For this review, use the dimensioned drawing (mm, ordinates from the lowest corner) and the shaded views. Round coordinates to 2 decimals unless told otherwise and drop trailing zeros. Write each loop counter-clockwise with the first axis right and the second up, starting at its lowest first coordinate (ties: lowest second). Pieces come first, ordered by that corner, then holes.
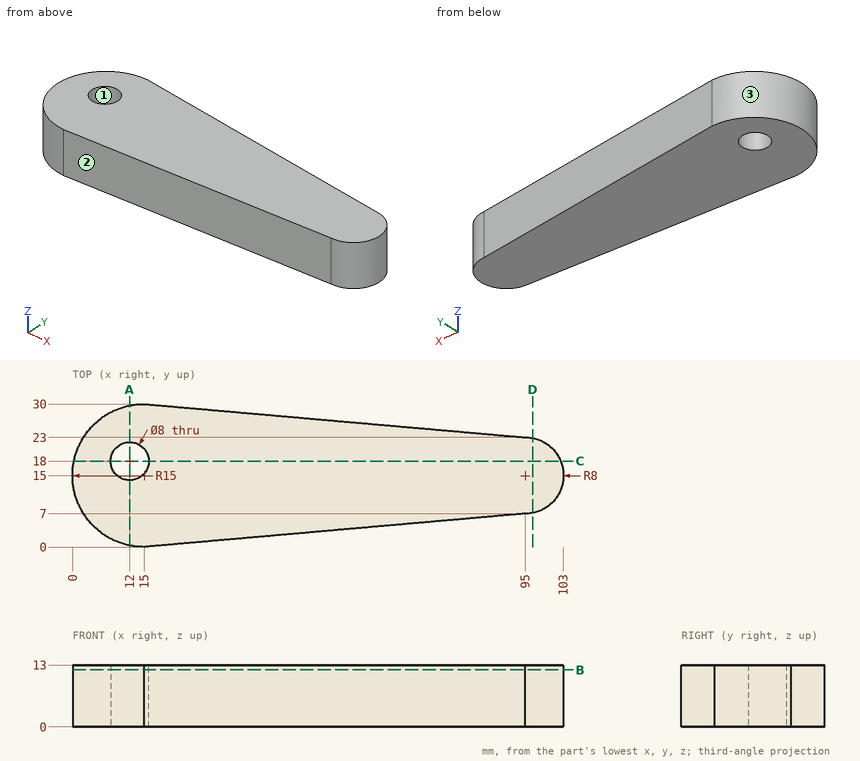
1) Add section C-C on y = 18. State the section outline as (x, z) points, and give its area (3 significant figures).
2) Add section A-A on x = 12. State the section outline as (y, z) points.
3) For line 1 along Y through (x, z) = (12, 7.25); line 2 along X through (y, z) = (18, 9.5); line 3 along X through (y, z) = (16.75, 4.75), list the stretches that pass through material, from the lowest coordinate up.
4) For P1, Ø2, axis at y = 20.5, z = 2.5, coming from the +X side; P2, Ø1, axis at y = 20, z = 6.5, coming from the -X side, all flat-tipped, find the tip position at first contact; note any pin that passes through.
5) Add section B-B on z = 12. State the section outline as (x, y) points, and give its area (3 significant figures).
6) The part is to be moulded in two halves that separate along X. For the marked faces 1, 2 and 3, say which applies: pulls with the +X half, pulls with the -X half, needs draft (parallel to the pull), parting line crosses it, or undercut.
7) Add section D-D on x = 96.5. State the section outline as (y, z) points, and give its area (3 significant figures).
Computed:
1. outline: (0.3, 0) - (8, 0) - (8, 13) - (0.3, 13) - close; (16, 0) - (102.42, 0) - (102.42, 13) - (16, 13) - close
1. area: 1,220 mm2
2. outline: (0.3, 0) - (14, 0) - (14, 13) - (0.3, 13) - close; (22, 0) - (29.7, 0) - (29.7, 13) - (22, 13) - close
3. line 1: y = 0.3 to 14, 22 to 29.7
3. line 2: x = 0.3 to 8, 16 to 102.42
3. line 3: x = 0.1 to 8.2, 15.8 to 102.81
4. P1: stops at x = 101.61
4. P2: stops at x = 0.69
5. outline: (15, 0) - (95, 7) arc R8 ccw to (95, 23) - (15, 30) arc R15 ccw to start; hole circle Ø8 at (12, 18)
5. area: 2,240 mm2
6. face 1: undercut
6. face 2: pulls with the +X half
6. face 3: pulls with the -X half
7. outline: (7.14, 0) - (22.86, 0) - (22.86, 13) - (7.14, 13) - close
7. area: 204 mm2
